from build123d import *

# Parameters (mm, degrees)
ESBO_O2_R             = 12.75
ESBO_O2_R_2           = 10.75
ESBO_O3_R             = 16
CORTE_EXTRUS_O1_DEPTH = 35


with BuildPart() as part:
    # Varredura1: sweep along a path in Esboço1
    with BuildLine(Plane.XY) as varredura1_path:
        Line((-193.129443739, 25.425973626), (-6.526309611, 0.85920496))
        ThreePointArc((-6.526309611, 0.85920496), (0, 0.431448029), (6.526309611, 0.85920496))
        Line((6.526309611, 0.85920496), (191.870520585, 25.260233248))
    # Esboço2 → Varredura1 (sweep)
    with BuildSketch(Plane(origin=(191.870520585, 25.260233248, 0), x_dir=(0, 0, -1), z_dir=(0.9914448613738109, 0.13052619222004852, 0))):
        Circle(ESBO_O2_R)
        Circle(ESBO_O2_R_2, mode=Mode.SUBTRACT)
    sweep(path=varredura1_path.line)

    # Esboço3 → Corte-extrusão1 (cut, symmetric)
    with BuildSketch(Plane.XY):
        with Locations((-202.713054604, 26.687679932)):
            Circle(ESBO_O3_R)
    corte_extrus_o1 = extrude(amount=CORTE_EXTRUS_O1_DEPTH, both=True, mode=Mode.SUBTRACT)

    # Espelhar1: Corte-extrusão1 across plane
    add(corte_extrus_o1.mirror(Plane(origin=(0, 0, 0), x_dir=(0, 0, 1), z_dir=(1, 0, 0))), mode=Mode.SUBTRACT)


solid = part.part
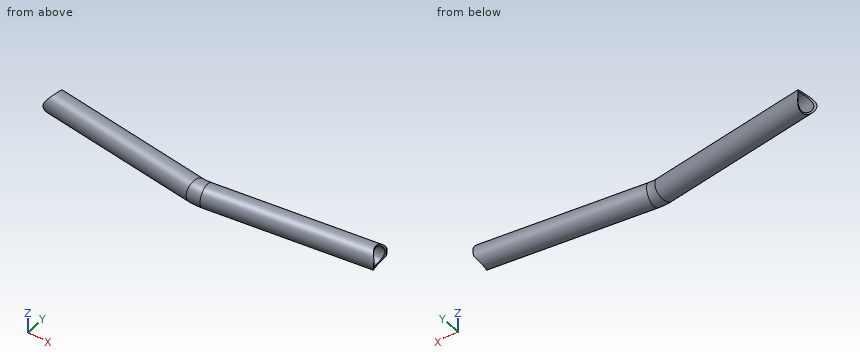
Geometry check sheet. Reference: the model listing, model coordinates, mm. Give positions to 0.01 mm unless a question says otherwise; leave off trailing zeros. Order: outer loops, then holes, each group sorted by start corner. A loop starts at its lowest first (then second) coordinate and runs counter-clockwise, first axis right, second up. Notation, with made-up numbers: (88, 37) - (147, 37) arc R18 ccw to (147, 49) - close; hole circle Ø5 at (-33, 75.5). An arc over 180 degrees is marked (long way). Use one line per item in the form item = value.
1) Depth check by flat-ended pin: pin 1 Ø2 at (x, z) = (-88.5, -8) entering from +Y; pin 2 Ø3 at (x, z) = (54.5, 0.5) entering from -Y; pin 3 Ø3 at (x, y) = (-128.5, 23) entering from -Z. Enter the tip coordinate at first touch or a pass-through.
Working result:
pin_1 = 22.41
pin_2 = -5.88
pin_3 = -11.92
2) Sectioned sample at A-A (z = 0.75). Record the boundary of the cut face in (x, y).
Working result:
outline = (-194.76, 12.8) - (-8.19, -11.76) arc R62.73 ccw to (8.19, -11.76) - (193.53, 12.64) - (193.39, 13.68) arc R16 cw to (192.34, 14.51) - (7.93, -9.77) arc R60.72 cw to (-7.93, -9.77) - (-192.34, 14.51) arc R16 cw to start; (-191.44, 38.04) arc R16 cw to (-189.54, 35.77) - (-5.13, 11.49) arc R39.28 ccw to (5.13, 11.49) - (189.54, 35.77) arc R16 cw to (190.35, 36.84) - (190.21, 37.88) - (4.86, 13.48) arc R37.27 cw to (-4.86, 13.48) - close
3) Material ranges on probe 1 along Z at (x, y) = (138.5, 17.5); probe 2 along Z at (x, y) = (32.5, 13); probe 3 along Y at (x, z) = (162.5, 7) (3 decimals), recorded low to high. Write a range as from..to.
Working result:
probe_1 = -12.73..-10.73, 10.73..12.73
probe_2 = -9.37..-6.39, 6.39..9.37
probe_3 = 10.645..13.165, 29.623..32.142
